```python
from build123d import *

# Parameters (mm, degrees)
SKETCH_W      = 25
SKETCH_H      = 15
PAD_DEPTH     = 5
PAD001_DEPTH  = 16
SKETCH002_R   = 2.5
POCKET_DEPTH  = 15
SKETCH003_R   = 10.5
SKETCH003_R_2 = 7.5
PAD002_DEPTH  = 20
SKETCH004_W   = 55.5
SKETCH004_H   = 21
SKETCH004_R   = 7.5
PAD003_DEPTH  = 3
SKETCH005_W   = 3
SKETCH005_H   = 21
PAD004_DEPTH  = 14


with BuildPart() as part:
    # Sketch → Pad (new body)
    with BuildSketch(Plane.XY):
        with BuildLine():
            Line((0, -35.5), (0, 27.5))
            Line((0, 27.5), (50.5, 27.5))
            ThreePointArc((55.5, 22.5), (54.035534, 26.035534), (50.5, 27.5))
            Line((55.5, 22.5), (55.5, 0))
            Line((55.5, 0), (10, 0))
            Line((10, 0), (10, -25.5))
            Line((10, -25.5), (55.5, -25.5))
            Line((55.5, -25.5), (55.5, -35.5))
            Line((55.5, -35.5), (0, -35.5))
        make_face()
        with Locations((30.25, 11.25)):
            Rectangle(SKETCH_W, SKETCH_H, mode=Mode.SUBTRACT)
    extrude(amount=PAD_DEPTH)

    # Sketch001 (on Face15 of Pad) → Pad001 (join)
    with BuildSketch(Plane.XY.offset(5)):
        with BuildLine():
            Line((55.5, 22.5), (55.5, 0))
            Line((55.5, 0), (50.5, 0))
            Line((50.5, 0), (50.5, 22.5))
            Line((50.5, 22.5), (10, 22.5))
            Line((10, 22.5), (10, -25.5))
            Line((55.5, -25.5), (10, -25.5))
            Line((55.5, -35.5), (55.5, -25.5))
            Line((0, -35.5), (55.5, -35.5))
            Line((0, 27.5), (0, -35.5))
            Line((50.5, 27.5), (0, 27.5))
            ThreePointArc((55.5, 22.5), (54.035534, 26.035534), (50.5, 27.5))
        make_face()
    extrude(amount=PAD001_DEPTH)

    # Sketch002 (on Face26 of Pad001) → Pocket (cut)
    with BuildSketch(Plane.XZ.offset(35.5)):
        with Locations((27.75, 10.5)):
            Circle(SKETCH002_R)
    extrude(amount=-POCKET_DEPTH, mode=Mode.SUBTRACT)

    # Sketch003 (on Face26 of Pocket) → Pad002 (join)
    with BuildSketch(Plane.XZ.offset(35.5)):
        with Locations((27.75, 10.5)):
            Circle(SKETCH003_R)
        with Locations((27.75, 10.5)):
            Circle(SKETCH003_R_2, mode=Mode.SUBTRACT)
    extrude(amount=PAD002_DEPTH)

    # Sketch004 (on Face32 of Pad002) → Pad003 (join)
    with BuildSketch(Plane.XZ.offset(55.5)):
        with Locations((27.75, 10.5)):
            Rectangle(SKETCH004_W, SKETCH004_H)
        with Locations((27.75, 10.5)):
            Circle(SKETCH004_R, mode=Mode.SUBTRACT)
    extrude(amount=PAD003_DEPTH)

    # Sketch005 (on Face33 of Pad003) → Pad004 (join)
    with BuildSketch(Plane(origin=(0, -55.5, 0), x_dir=(-1, 0, 0), z_dir=(0, 1, 0))):
        with Locations((-54, 10.5)):
            Rectangle(SKETCH005_W, SKETCH005_H)
        with Locations((-1.5, 10.5)):
            Rectangle(SKETCH005_W, SKETCH005_H)
    extrude(amount=PAD004_DEPTH)


solid = part.part
```
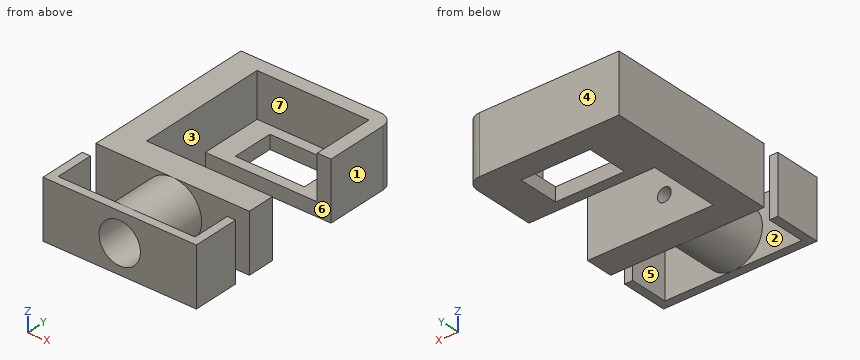
Here's how the part is built. I have some questions about the finished solid (model axes, mm). Face numbers are marked on the shaded views. A direction names the side the tool comes from. Give positions to 0.01 mm unless a question says otherwise; leave off trailing zeros. Loops run counter-clockwise (first coordinate to the right, second up) from the corner with the lowest first, then second, coordinate; pieces in that order, holes last. Notation, with made-up numbers: M 20.25,58 L 74.25,58 A15 ccw 74.25,84 Z; hole C -9.75,3.25 d1. An arc over 180 degrees is marked long. Put each result on its own line as item: value. Start each with the question number.
(1) Will these pins go through, and if not, where does the flat tip stop? pin 1 Ø4.5 at (x, z) = (26.5, 11) entering from -Y; pin 2 Ø1 at (y, z) = (-39.5, 13.5) entering from -X; pin 3 Ø3 at (y, z) = (-17, 8) entering from +X.
(2) For the marked faces 5, 6 and 7, which set-ups out of +Z, -Z, +X, -X, +Y, -Y let a thin tool reach every point of the face, with its end or its side?
(3) I need wall thicknesses on line 1 along Y through (x, z) = (23, 20.25); line 2 along Y through (x, z) = (12, 3); line 3 along Y through (x, z) = (42.5, 4.5). Which ranges of each line are inside material? Lowest first, please. Write a range as [from, to].
(4) If we mould it in two halves opening along Y, with no side actions, what happens to the marked faces 1, 2, 3 and 4? For each: +Y half, -Y half, draft (parallel to the pull), parting line (faces both ways), or undercut.
(5) I want a section at C-C on y = -31. Please give me the cut outline in (x, z).
(6) I want a section at B-B on y = 17. Please give me the cut outline in (x, z).
(7) I want a section at D-D on x = 33.5. Please give me the cut outline in (y, z), then the cut area to 3 significant figures.
Answer block:
1. pin 1: y = -35.5
1. pin 2: x = 17.55
1. pin 3: x = 10
2. face 5: +Z, -Z
2. face 6: +Z, -Z, +X
2. face 7: +Z
3. line 1: [-58.5, -55.5], [-35.5, -25.5], [22.5, 27.5]
3. line 2: [-58.5, -55.5], [-35.5, -25.5], [0, 27.5]
3. line 3: [-58.5, -55.5], [-35.5, -25.5], [0, 3.75], [18.75, 27.5]
4. face 1: draft
4. face 2: undercut
4. face 3: undercut
4. face 4: +Y half
5. outline: M 0,0 L 55.5,0 L 55.5,21 L 0,21 Z; hole C 27.75,10.5 d5
6. outline: M 0,0 L 17.75,0 L 17.75,5 L 10,5 L 10,21 L 0,21 Z; M 42.75,0 L 55.5,0 L 55.5,21 L 50.5,21 L 50.5,5 L 42.75,5 Z
7. outline: M -58.5,0 L -55.5,0 L -55.5,1.71 L -35.5,1.71 L -35.5,0 L -25.5,0 L -25.5,21 L -35.5,21 L -35.5,19.29 L -55.5,19.29 L -55.5,21 L -58.5,21 L -58.5,15.32 L -35.5,15.32 L -35.5,5.68 L -58.5,5.68 Z; M 0,0 L 3.75,0 L 3.75,5 L 0,5 Z; M 18.75,0 L 27.5,0 L 27.5,21 L 22.5,21 L 22.5,5 L 18.75,5 Z
7. area: 545 mm^2
